```python
from build123d import *

# Parameters (mm, degrees)
BOSS_EXTRUDE1_DEPTH = 327.5
SKETCH7_W           = 83
SKETCH7_H           = 2
CUT_EXTRUDE7_DEPTH  = 203
SKETCH2_R           = 1.6
CUT_EXTRUDE2_DEPTH  = 10
SKETCH3_R           = 1.93
CUT_EXTRUDE3_DEPTH  = 102
SKETCH4_R           = 1.93
CUT_EXTRUDE4_DEPTH  = 10
SKETCH5_W           = 130.251709281
SKETCH5_H           = 163.75
CUT_EXTRUDE6_DEPTH  = 231


with BuildPart() as part:
    # Sketch1 → Boss-Extrude1 (new body)
    with BuildSketch(Plane(origin=(0, 0, 0), x_dir=(1, 0, 0), z_dir=(0, 1, 0))):
        Polygon((0, -0.603), (0, 101.206), (101.206, 101.206), (101.206, -0.6), (91.5, -0.6), (91.5, 1.4), (85.703, 1.4), (85.703, 3.4), (93.5, 3.4), (93.5, 2), (99.206, 2), (99.206, 99.206), (2, 99.206), (2, 2), (7.706, 2), (7.706, 3.397), (15.503, 3.397), (15.503, 1.397), (9.706, 1.397), (9.706, -0.603), align=None)
    extrude(amount=BOSS_EXTRUDE1_DEPTH)

    # Sketch7 → Cut-Extrude7 (cut)
    with BuildSketch(Plane(origin=(0, 327.5, 0), x_dir=(1, 0, 0), z_dir=(0, 1, 0))):
        with Locations((50.603, 0.397)):
            Rectangle(SKETCH7_W, SKETCH7_H)
    extrude(amount=-CUT_EXTRUDE7_DEPTH, mode=Mode.SUBTRACT)

    # Sketch2 → Cut-Extrude2 (cut)
    with BuildSketch(Plane.XY.offset(-1.397)):
        with Locations((12.303, 314.9)):
            Circle(SKETCH2_R)
        with Locations((12.303, 308.5)):
            Circle(SKETCH2_R)
        with Locations((88.903, 314.9)):
            Circle(SKETCH2_R)
        with Locations((88.903, 308.5)):
            Circle(SKETCH2_R)
        with Locations((12.303, 240.925)):
            Circle(SKETCH2_R)
        with Locations((12.303, 234.525)):
            Circle(SKETCH2_R)
        with Locations((88.903, 240.925)):
            Circle(SKETCH2_R)
        with Locations((88.903, 234.525)):
            Circle(SKETCH2_R)
        with Locations((12.303, 166.95)):
            Circle(SKETCH2_R)
        with Locations((12.303, 160.55)):
            Circle(SKETCH2_R)
        with Locations((88.903, 166.95)):
            Circle(SKETCH2_R)
        with Locations((88.903, 160.55)):
            Circle(SKETCH2_R)
        with Locations((12.303, 92.975)):
            Circle(SKETCH2_R)
        with Locations((12.303, 86.575)):
            Circle(SKETCH2_R)
        with Locations((88.903, 92.975)):
            Circle(SKETCH2_R)
        with Locations((88.903, 86.575)):
            Circle(SKETCH2_R)
        with Locations((12.303, 19)):
            Circle(SKETCH2_R)
        with Locations((12.303, 12.6)):
            Circle(SKETCH2_R)
        with Locations((88.903, 19)):
            Circle(SKETCH2_R)
        with Locations((88.903, 12.6)):
            Circle(SKETCH2_R)
    extrude(amount=-CUT_EXTRUDE2_DEPTH, mode=Mode.SUBTRACT)

    # Sketch3 → Cut-Extrude3 (cut)
    with BuildSketch(Plane(origin=(101.206, 0, 0), x_dir=(0, 0, -1), z_dir=(1, 0, 0))):
        with Locations((50.603, 322.524)):
            Circle(SKETCH3_R)
        with Locations((50.603, 4.976)):
            Circle(SKETCH3_R)
    extrude(amount=-CUT_EXTRUDE3_DEPTH, mode=Mode.SUBTRACT)

    # Sketch4 → Cut-Extrude4 (cut)
    with BuildSketch(Plane(origin=(0, 0, -101.206), x_dir=(-1, 0, 0), z_dir=(0, 0, -1))):
        with Locations((-50.603, 322.524)):
            Circle(SKETCH4_R)
        with Locations((-50.603, 4.976)):
            Circle(SKETCH4_R)
    extrude(amount=-CUT_EXTRUDE4_DEPTH, mode=Mode.SUBTRACT)

    # Sketch5 → Cut-Extrude6 (cut)
    with BuildSketch(Plane.ZY):
        with Locations((-36.08014536, 81.875)):
            Rectangle(SKETCH5_W, SKETCH5_H)
    extrude(amount=-CUT_EXTRUDE6_DEPTH, mode=Mode.SUBTRACT)


solid = part.part
```
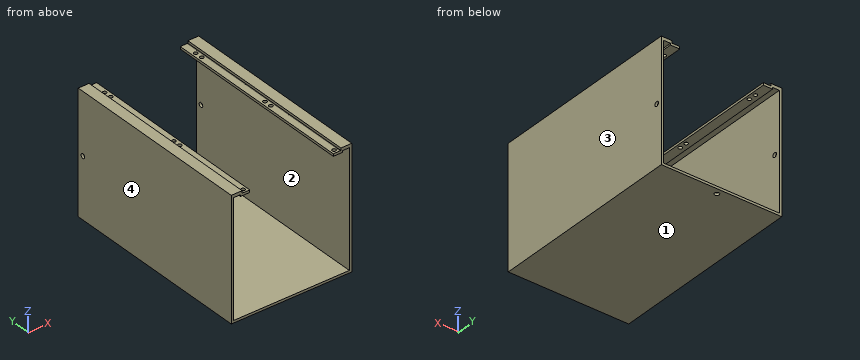
CAD build for the part. Positions are in the model's coordinates, mm. Face numbers are marked on the shaded views. Round coordinates to 2 decimals unless told otherwise and drop trailing zeros. Order: outer loops, then holes, each group sorted by start corner. A loop starts at its lowest first (then second) coordinate and runs counter-clockwise, first axis right, second up.
Q1. Two-plate mould, pull along X, no slides. Class the marked faces 1, 2, 3 and 4: pulls with the +X half, pulls with the -X half, needs draft (parallel to the pull), parting line crosses it, or undercut.
Q2. Wall check: L1, parallel to X at y = 252, z = -51; L2, parallel to Z at x = 8, y = 236; L3, parallel to Z at x = 97.5, y = 238. Give the ranges that are in metal, low to high.
Q3. Slice it at C-C (x = 73). Write the cut outline in (y, z).
Q4. Drop flat-ended pins along their axis: pin 1 (5 mm diameter, centred on x = 12.303, y = 234.525, fed in from +Z); pin 2 (1.9 mm diameter, centred on x = 88.903, y = 166.95, fed in from +Z); pin 3 (10 mm diameter, centred on x = 96, y = 262.5, fed in from +Z). Give the stop position or say it passes through.
Q5. Slice it at A-A (z = -45.5). Write the cut outline in (x, y), and give its area (3 significant figures).
Results below:
1. face 1: needs draft
1. face 2: undercut
1. face 3: pulls with the +X half
1. face 4: pulls with the -X half
2. L1: x = 0 to 2, 99.21 to 101.21
2. L2: z = -101.21 to -99.21, -3.4 to 0.6
2. L3: z = -101.21 to -99.21, -2 to 0.6
3. outline: (163.75, -101.21) - (327.5, -101.21) - (327.5, -99.21) - (163.75, -99.21) - close
4. pin 1: stops at z = -1.4
4. pin 2: stops at z = -99.21
4. pin 3: stops at z = 0.6
5. outline: (0, 163.75) - (2, 163.75) - (2, 327.5) - (0, 327.5) - close; (99.21, 163.75) - (101.21, 163.75) - (101.21, 327.5) - (99.21, 327.5) - close
5. area: 655 mm2
